Read the model definition and answer for the solid it produces. Units are mm, in the model's axes. A direction names the side the tool comes from. Round coordinates to 2 decimals unless told otherwise and drop trailing zeros. Write each loop counter-clockwise with the first axis right and the second up, starting at its lowest first coordinate (ties: lowest second). Pieces come first, ordered by that corner, then holes. Notation, with made-up numbers: (-11.5, -9.5) -> (11.5, -9.5) arc R30 ccw to (11.5, 21.5) -> close; hole circle Ø2 at (-29.5, 80). An arc over 180 degrees is marked (long way). Return JSON: item names as keys, results as strings. Group by question number.
(1) Straight lines are drawn through the part: line 1 (X direction, y = 20.5, z = 7); line 2 (X direction, y = 145, z = 1.25); line 3 (Y direction, x = 42, z = 8.5). For each, find the intervals that lie inside material, in ascending order.
(2) A cutting plane is placed at C-C on x = 80. Give the vertices of the cut face in (y, z), then the cut area to 3 significant figures.
(3) A cutting plane is placed at A-A on y = 20. Give the vertices of the cut face in (x, z).
(4) The mould has two halves that part along X. Classify faces 1 (the flat face through (0, 66, 5)), 2 (the flat face through (44, -30, 5)), 3 (the flat face through (120.526, 78, 5)): released by +X, released by -X, zero draft, split by the parting line, or undercut.
(5) For faces 4 (the flat face through (-29.474, 78, 5)), 5 (the flat face through (32, 129, 5)), determine the directions among +Z, -Z, +X, -X, +Y, -Y from which every point of the face is accessible in a straight line to the end or side of a thin tool.
(6) A cutting plane is placed at B-B on z = 5.5. Give the vertices of the cut face in (x, y), then the cut area to 3 significant figures.
```python
from build123d import *

# Parameters (mm, degrees)
F1_W     = 150
F1_H     = 220
F2_DEPTH = 10
F3_DEPTH = 25


with BuildPart() as f2:
    # F1 (on Top) → F2 (new body)
    with BuildSketch(Plane.XY):
        with Locations((45.525713, 80)):
            Rectangle(F1_W, F1_H)
    extrude(amount=F2_DEPTH)

    # F0 (on Top) → F3 (cut)
    with BuildSketch(Plane.XY):
        Polygon((14.999021, 7), (10.525713, 0), (83.010264, 0), (75.500965, 7), align=None)
        Polygon((25, 120), (0, 120), (0, 10.580182), (7, 15.109896), (7, 113), (32, 113), (32, 146.241054), (25, 152.102575), align=None)
        Polygon((83, 14.64067), (90, 9.280561), (90, 120), (65, 120), (65, 152.879447), (58, 146.40218), (58, 113), (83, 113), align=None)
        Polygon((57.524528, 160), (31.603869, 160), (36.329959, 153), (53.748887, 153), align=None)
    extrude(amount=F3_DEPTH, mode=Mode.SUBTRACT)


solid = f2.part
```
Checks:
{
 "1": {"line 1": "x = -29.47 to 0, 7 to 83, 90 to 120.53", "line 2": "x = -29.47 to 25, 32 to 58, 65 to 120.53", "line 3": "y = -30 to 0, 7 to 153, 160 to 190"},
 "2": {"outline": "(-30, 0) -> (0, 0) -> (0, 10) -> (-30, 10) -> close; (2.81, 0) -> (113, 0) -> (113, 10) -> (2.81, 10) -> close; (120, 0) -> (190, 0) -> (190, 10) -> (120, 10) -> close", "area": "2,100 mm^2"},
 "3": {"outline": "(-29.47, 0) -> (0, 0) -> (0, 10) -> (-29.47, 10) -> close; (7, 0) -> (83, 0) -> (83, 10) -> (7, 10) -> close; (90, 0) -> (120.53, 0) -> (120.53, 10) -> (90, 10) -> close"},
 "4": {"face 1": "undercut", "face 2": "zero draft", "face 3": "released by +X"},
 "5": {"face 4": "+Z, -Z, -X, +Y, -Y", "face 5": "+Z, -Z"},
 "6": {"outline": "(-29.47, -30) -> (120.53, -30) -> (120.53, 190) -> (-29.47, 190) -> close; hole (0, 10.58) -> (7, 15.11) -> (7, 113) -> (32, 113) -> (32, 146.24) -> (25, 152.1) -> (25, 120) -> (0, 120) -> close; hole (10.53, 0) -> (83.01, 0) -> (75.5, 7) -> (15, 7) -> close; hole (31.6, 160) -> (36.33, 153) -> (53.75, 153) -> (57.52, 160) -> close; hole (58, 113) -> (83, 113) -> (83, 14.64) -> (90, 9.28) -> (90, 120) -> (65, 120) -> (65, 152.88) -> (58, 146.4) -> close", "area": "30,100 mm^2"}
}
